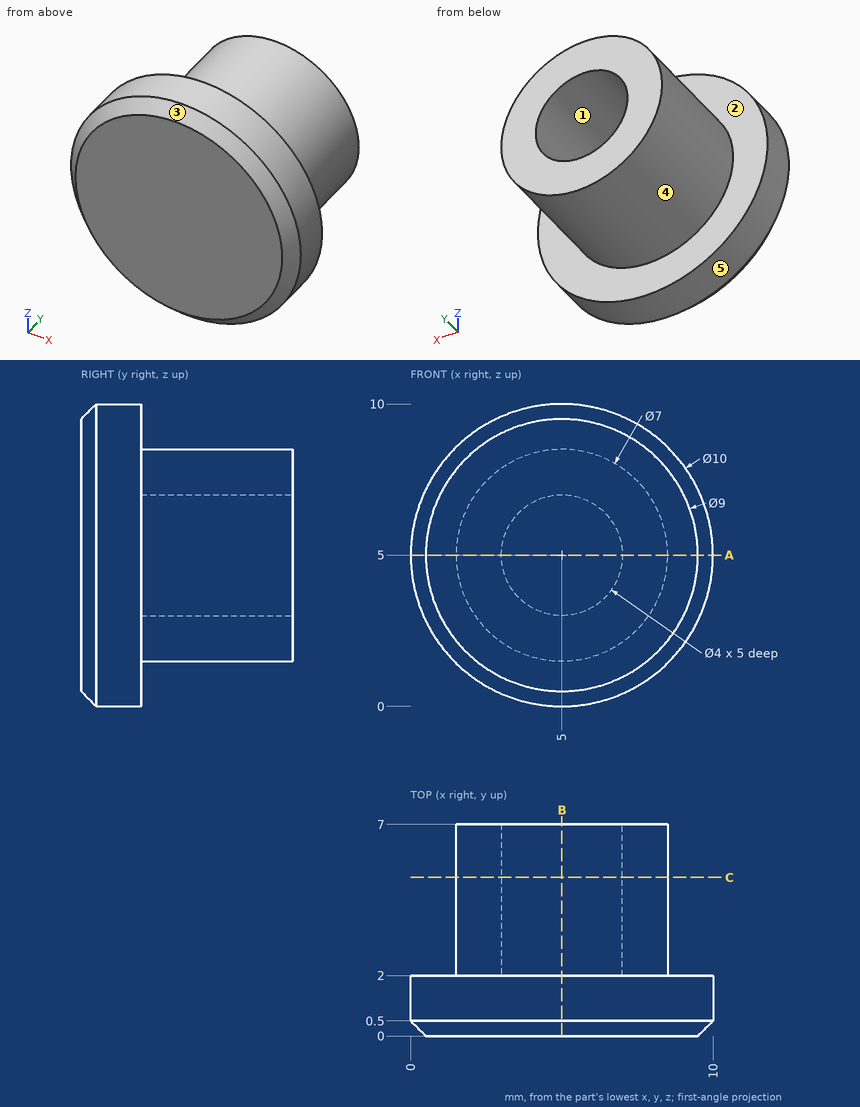
Design review of the part shown in the three views and the two pictorial views. Dimensions are in mm from the part's minimum x, y and z. A direction names the side the tool comes from. Round coordinates to 2 decimals unless told otherwise and drop trailing zeros. Write each loop counter-clockwise with the first axis right and the second up, starting at its lowest first coordinate (ties: lowest second). Pieces come first, ordered by that corner, then holes. Notation, with made-up numbers: (40, -38.75) -> (70, -38.75) arc R33 ccw to (70, -5.75) -> close; hole circle Ø8 at (-22.75, 10). An arc over 180 degrees is marked (long way). One line per question, with ' | ' between items. Start each with the question number.
1) Machinability: for the marked faces 4 and 5, which of the approach directions +Z, -Z, +X, -X, +Y, -Y give a long, thin tool a straight path to every point of the face, cutting with its end or side? Answer none if there is none.
2) Add section A-A (z = 5). Write out the cut boundary in (x, y).
3) Wall thickness on line 1 along Z through (x, y) = (5, 3.35); line 2 along Y through (x, z) = (4.75, 6.75); line 3 along Z through (x, y) = (3.5, 4): over which ranges is each line inside the solid? List them lowest first.
4) Mouldability with a two-part tool opening along X and no side actions: class the marked faces 1, 2 and 3 as +X half, -X half, draft (parallel to the pull), parting line (faces both ways), or undercut.
5) Add section B-B (x = 5). Write out the cut boundary in (y, z).
6) Add section C-C (y = 5.25). Write out the cut boundary in (x, z), and give its area (3 significant figures).
7) For pin 1 Ø1.5 at (x, y) = (7, 4.5) entering from +Z; pin 2 Ø2 at (x, y) = (7, 4.5) entering from -Z; pin 3 Ø1.5 at (x, z) = (5, 5) entering from +Y; pin 4 Ø5 at (x, z) = (5.5, 4.5) entering from +Y, all flat-tipped, find the tip position at first contact; note any pin that passes through.
Reported:
1) face 4: +Y | face 5: +Y, -Y
2) outline: (0, 0.5) -> (0.5, 0) -> (9.5, 0) -> (10, 0.5) -> (10, 2) -> (8.5, 2) -> (8.5, 7) -> (7, 7) -> (7, 2) -> (3, 2) -> (3, 7) -> (1.5, 7) -> (1.5, 2) -> (0, 2) -> close
3) line 1: z = 1.5 to 3, 7 to 8.5 | line 2: y = 0 to 2 | line 3: z = 1.84 to 3.68, 6.32 to 8.16
4) face 1: undercut | face 2: draft | face 3: parting line
5) outline: (0, 0.5) -> (0.5, 0) -> (2, 0) -> (2, 1.5) -> (7, 1.5) -> (7, 3) -> (2, 3) -> (2, 7) -> (7, 7) -> (7, 8.5) -> (2, 8.5) -> (2, 10) -> (0.5, 10) -> (0, 9.5) -> close
6) outline: circle Ø7 at (5, 5); hole circle Ø4 at (5, 5) | area: 25.9 mm²
7) pin 1: stops at z = 8.27 | pin 2: stops at z = 1.65 | pin 3: stops at y = 2 | pin 4: stops at y = 7
